from build123d import *

# Parameters (mm, degrees)
SKETCH1_W           = 95
SKETCH1_H           = 150
SKETCH1_W_2         = 90
SKETCH1_H_2         = 145
BOSS_EXTRUDE1_DEPTH = 2.5
BOSS_EXTRUDE2_DEPTH = 5
FILLET1_R           = 2.5
CHAMFER1_SIZE       = 0.5


with BuildPart() as part:
    # Sketch1 → Boss-Extrude1 (new body)
    # profile 1 of 2: a face of its own
    with BuildSketch(Plane(origin=(0, 0, 0), x_dir=(1, 0, 0), z_dir=(0, 1, 0))):
        with Locations((0, 75)):
            Rectangle(SKETCH1_W, SKETCH1_H)
        with Locations((0, 75)):
            Rectangle(SKETCH1_W_2, SKETCH1_H_2, mode=Mode.SUBTRACT)
    # profile 2 of 2: a face of its own
    with BuildSketch(Plane(origin=(0, 0, 0), x_dir=(1, 0, 0), z_dir=(0, 1, 0))):
        with Locations((0, 75)):
            Rectangle(SKETCH1_W_2, SKETCH1_H_2)
    extrude(amount=BOSS_EXTRUDE1_DEPTH)

    # Sketch2 → Boss-Extrude2 (add)
    with BuildSketch(Plane(origin=(0, 2.5, 0), x_dir=(1, 0, 0), z_dir=(0, 1, 0))):
        Polygon((-19, 8.5), (-19, 3.5), (-44, 3.5), (-44, 28.5), (-39, 28.5), (-39, 8.5), align=None)
        Polygon((19, 3.5), (19, 8.5), (39, 8.5), (39, 28.5), (44, 28.5), (44, 3.5), align=None)
        Polygon((-44, 146.5), (-44, 121.5), (-39, 121.5), (-39, 141.5), (-19, 141.5), (-19, 146.5), align=None)
        Polygon((39, 121.5), (44, 121.5), (44, 146.5), (19, 146.5), (19, 141.5), (39, 141.5), align=None)
    extrude(amount=BOSS_EXTRUDE2_DEPTH)

    # Fillet1
    fillet1_edges = [part.edges().sort_by_distance(p)[0] for p in [
        (47.5, 1.25, -150),
        (47.5, 1.25, 0),
        (-47.5, 1.25, 0),
        (-47.5, 1.25, -150),
        (44, 5, -146.5),
        (19, 5, -146.5),
        (19, 5, -141.5),
        (39, 5, -141.5),
        (39, 5, -121.5),
        (44, 5, -121.5),
        (-19, 5, -8.5),
        (-39, 5, -8.5),
        (-39, 5, -28.5),
        (-44, 5, -28.5),
        (-44, 5, -3.5),
        (-19, 5, -3.5),
        (-19, 5, -146.5),
        (-44, 5, -121.5),
        (-39, 5, -121.5),
        (-39, 5, -141.5),
        (-19, 5, -141.5),
        (19, 5, -3.5),
        (44, 5, -3.5),
        (44, 5, -28.5),
        (39, 5, -28.5),
        (39, 5, -8.5),
        (19, 5, -8.5),
        (-44, 5, -146.5),
    ]]
    fillet(fillet1_edges, radius=FILLET1_R - 0.0001)  # a hair under: the kernel refuses the full size

    # Chamfer1
    chamfer1_edges = [part.edges().sort_by_distance(p)[0] for p in [
        (-47.5, 2.5, -75),
        (0, 2.5, 0),
        (-46.767796242, 2.5, -149.267796242),
        (-46.767796242, 2.5, -0.732203758),
        (46.767796242, 2.5, -0.732203758),
        (46.767796242, 2.5, -149.267796242),
        (31.5, 7.5, -146.5),
        (44, 7.5, -134),
        (29, 7.5, -141.5),
        (39, 7.5, -131.5),
        (43.267796242, 7.5, -122.232203758),
        (39.732203758, 7.5, -122.232203758),
        (19.732203758, 7.5, -142.232203758),
        (19.732203758, 7.5, -145.767796242),
        (43.267796242, 7.5, -145.767796242),
        (-29, 7.5, -8.5),
        (-39, 7.5, -18.5),
        (-44, 7.5, -16),
        (-31.5, 7.5, -3.5),
        (-19.732203758, 7.5, -4.232203758),
        (-19.732203758, 7.5, -7.767796242),
        (-43.267796242, 7.5, -4.232203758),
        (-43.267796242, 7.5, -27.767796242),
        (-39.732203758, 7.5, -27.767796242),
        (-31.5, 7.5, -146.5),
        (-44, 7.5, -134),
        (-39, 7.5, -131.5),
        (-29, 7.5, -141.5),
        (-43.267796242, 7.5, -145.767796242),
        (-19.732203758, 7.5, -142.232203758),
        (-19.732203758, 7.5, -145.767796242),
        (-39.732203758, 7.5, -122.232203758),
        (-43.267796242, 7.5, -122.232203758),
        (31.5, 7.5, -3.5),
        (44, 7.5, -16),
        (39, 7.5, -18.5),
        (29, 7.5, -8.5),
        (19.732203758, 7.5, -7.767796242),
        (19.732203758, 7.5, -4.232203758),
        (39.732203758, 7.5, -27.767796242),
        (43.267796242, 7.5, -27.767796242),
        (43.267796242, 7.5, -4.232203758),
        (38.267796242, 7.5, -140.767796242),
        (-38.267796242, 7.5, -9.232203758),
        (-38.267796242, 7.5, -140.767796242),
        (38.267796242, 7.5, -9.232203758),
        (0, 0, -150),
        (0, 2.5, -150),
        (47.5, 0, -75),
        (0, 0, 0),
        (-47.5, 0, -75),
        (-46.767796242, 0, -149.267796242),
        (-46.767796242, 0, -0.732203758),
        (46.767796242, 0, -0.732203758),
        (46.767796242, 0, -149.267796242),
        (47.5, 2.5, -75),
    ]]
    chamfer(chamfer1_edges, length=CHAMFER1_SIZE)


solid = part.part
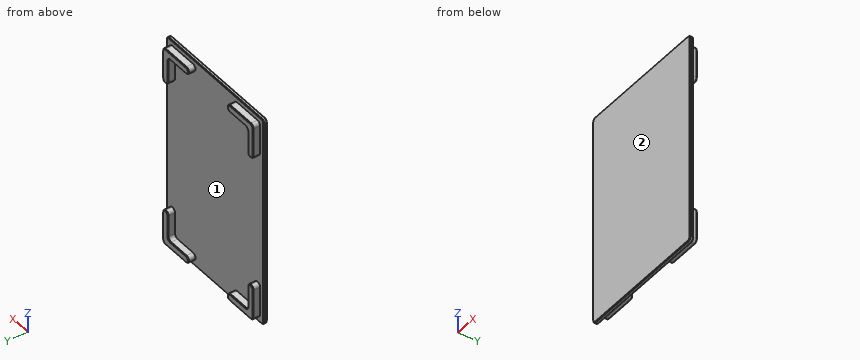
Could you check a few things on this model? Use its own coordinates, in mm. Face numbers are marked on the shaded views. Give positions to 0.01 mm unless a question says otherwise; leave off trailing zeros. Loops run counter-clockwise (first coordinate to the right, second up) from the corner with the lowest first, then second, coordinate; pieces in that order, holes last. Notation, with made-up numbers: (77, 58.25) -> (127, 58.25) arc R18 cw to (127, 88.25) -> close; hole circle Ø2 at (-6.75, 58.25). An arc over 180 degrees is marked (long way). Return JSON: item names as keys, results as strings.
Item 1: We'd pull the mould along X, two halves only. Please class the marked faces 1 and 2: +X half, -X half, draft (parallel to the pull), parting line (faces both ways), or undercut.
Geometry results:
{"face 1": "undercut", "face 2": "draft"}
Item 2: I'm going to push flat-ended pins straight in: pin 1 (3 mm diameter, centred on y = 4.5, z = -48, fed in from +X); pin 2 (2 mm diameter, centred on x = -31, y = 6, fed in from -Z); pin 3 (3.5 mm diameter, centred on y = 5, z = -132.5, fed in from -X); pin 4 (3.5 mm diameter, centred on y = 6, z = -18.5, fed in from +X). Where does each tip first touch, or does it pass through?
Geometry results:
{"pin 1": "passes through", "pin 2": "stops at z = -146.5", "pin 3": "stops at x = -44", "pin 4": "stops at x = 44"}
Item 3: I need wall thicknesses on L1, parallel to Z at x = 34, y = 3.5; L2, parallel to Y at x = 12, z = -137; L3, parallel to Z at x = 19.5, y = 5.25. Which ranges of each line are inside material? Lowest first, please. Write a range as from..to.
Geometry results:
{"L1": "z = -146.5..-141.5, -8.5..-3.5", "L2": "y = 0..2.5", "L3": "z = -145.5..-142.5, -7.5..-4.5"}
Item 4: If we section it at D-D on z = -128.5: List the corners of the cut face in (x, y) for me.
Geometry results:
{"outline": "(-47.5, 0.5) -> (-47, 0) -> (47, 0) -> (47.5, 0.5) -> (47.5, 2) -> (47, 2.5) -> (44, 2.5) -> (44, 7) -> (43.5, 7.5) -> (39.5, 7.5) -> (39, 7) -> (39, 2.5) -> (-39, 2.5) -> (-39, 7) -> (-39.5, 7.5) -> (-43.5, 7.5) -> (-44, 7) -> (-44, 2.5) -> (-47, 2.5) -> (-47.5, 2) -> close"}
Item 5: If we section it at C-C on x = -33: List the corners of the cut face in (y, z) for me.
Geometry results:
{"outline": "(0, -149.5) -> (0.5, -150) -> (2, -150) -> (2.5, -149.5) -> (2.5, -146.5) -> (7, -146.5) -> (7.5, -146) -> (7.5, -142) -> (7, -141.5) -> (2.5, -141.5) -> (2.5, -8.5) -> (7, -8.5) -> (7.5, -8) -> (7.5, -4) -> (7, -3.5) -> (2.5, -3.5) -> (2.5, -0.5) -> (2, 0) -> (0.5, 0) -> (0, -0.5) -> close"}
Item 6: If we section it at A-A on x = -3: List the corners of the cut face in (y, z) for me.
Geometry results:
{"outline": "(0, -149.5) -> (0.5, -150) -> (2, -150) -> (2.5, -149.5) -> (2.5, -0.5) -> (2, 0) -> (0.5, 0) -> (0, -0.5) -> close"}
Item 7: If we section it at B-B on z = -66: List the corners of the cut face in (x, y) for me, plus the area to 3 significant figures.
Geometry results:
{"outline": "(-47.5, 0.5) -> (-47, 0) -> (47, 0) -> (47.5, 0.5) -> (47.5, 2) -> (47, 2.5) -> (-47, 2.5) -> (-47.5, 2) -> close", "area": "237 mm²"}
